Work out the finished part from the listing and answer in its coordinate system (mm). A direction names the side the tool comes from. Round coordinates to 2 decimals unless told otherwise and drop trailing zeros. Order: outer loops, then holes, each group sorted by start corner. A loop starts at its lowest first (then second) coordinate and runs counter-clockwise, first axis right, second up. Notation, with made-up numbers: (19.25, -11.5) - (42.25, -11.5) arc R29 ccw to (42.25, 11.5) - close; hole circle Ø5 at (59, 0). An arc over 180 degrees is marked (long way). One line per question, with ' | ' between items. Start each with the question number.
from build123d import *

# Parameters (mm, degrees)
BOSS_EXTRUDE2_DEPTH      = 7
BOSS_EXTRUDE4_DEPTH      = 3
BOSS_EXTRUDE4_DEPTH_BACK = 3.4
SKETCH2_W                = 10
SKETCH2_H                = 10
SKETCH3_R                = 1.5
CUT_EXTRUDE1_DEPTH       = 10
SKETCH4_W                = 8
SKETCH4_H                = 3
BOSS_EXTRUDE5_DEPTH      = 7
SKETCH5_R                = 1.5
CUT_EXTRUDE2_DEPTH       = 7
FILLET1_R                = 5
FILLET2_R                = 5
FILLET3_R                = 5
FILLET4_R                = 2
FILLET5_R                = 2
SKETCH6_W                = 30
SKETCH6_H                = 41
BOSS_EXTRUDE6_DEPTH      = 8
SKETCH7_W                = 20
SKETCH7_H                = 23
CUT_EXTRUDE3_DEPTH       = 24
SKETCH8_R                = 1.5
CUT_EXTRUDE5_DEPTH       = 54


with BuildPart() as part:
    # Sketch1 → Boss-Extrude2 (new body)
    with BuildSketch(Plane.XY):
        with BuildLine():
            Line((36, 0), (31, 0))
            ThreePointArc((31, 0), (30.997217748, -0.415321451), (30.98887149, -0.830568352))
            ThreePointArc((30.98887149, -0.830568352), (29.746163614, -2.974229152), (30.539836631, -5.321501534))
            ThreePointArc((30.539836631, -5.321501534), (0.032857513, -30.999982587), (-30.528487289, -5.386229095))
            ThreePointArc((-30.528487289, -5.386229095), (-29.731741507, -3.029439038), (-30.987456583, -0.881779181))
            ThreePointArc((-30.987456583, -0.881779181), (-30.996863987, -0.440934196), (-31, 0))
            Line((-31, 0), (-36, 0))
            ThreePointArc((-36, 0), (-30.002092566, -19.89659372), (-14.006975463, -33.163302586))
            Line((-14.006975463, -33.163302586), (-14.006975463, -72.252490852))
            Line((-14.006975463, -72.252490852), (15.993024537, -72.252490852))
            Line((15.993024537, -72.252490852), (15.993024537, -32.252490852))
            ThreePointArc((15.993024537, -32.252490852), (30.592065012, -18.976974425), (36, 0))
        make_face()
    extrude(amount=BOSS_EXTRUDE2_DEPTH)

    # Sketch2 → Boss-Extrude4 (add, two sides: drawn at the far end of the back side and taken through both)
    with BuildSketch(Plane(origin=(0, 0, 0), x_dir=(-1, 0, 0), z_dir=(0, 0, -1)).offset(-BOSS_EXTRUDE4_DEPTH_BACK)):
        with Locations((38, 0)):
            Rectangle(SKETCH2_W, SKETCH2_H)
    extrude(amount=BOSS_EXTRUDE4_DEPTH + BOSS_EXTRUDE4_DEPTH_BACK)

    # Sketch3 → Cut-Extrude1 (cut)
    with BuildSketch(Plane.XY.offset(3.4)):
        with Locations((-39, 1)):
            Circle(SKETCH3_R)
    extrude(amount=-CUT_EXTRUDE1_DEPTH, mode=Mode.SUBTRACT)

    # Sketch4 → Boss-Extrude5 (add)
    with BuildSketch(Plane(origin=(0, 0, 0), x_dir=(-1, 0, 0), z_dir=(0, 0, -1))):
        with Locations((-39, -1.5)):
            Rectangle(SKETCH4_W, SKETCH4_H)
    extrude(amount=-BOSS_EXTRUDE5_DEPTH)

    # Sketch5 → Cut-Extrude2 (cut)
    with BuildSketch(Plane.XZ.offset(3)):
        with Locations((39.374782229, 3.5)):
            Circle(SKETCH5_R)
    extrude(amount=-CUT_EXTRUDE2_DEPTH, mode=Mode.SUBTRACT)

    # Fillet1
    fillet1_edges = [part.edges().sort_by_distance(p)[0] for p in [
        (-43, -5, 0.2),
    ]]
    fillet(fillet1_edges, radius=FILLET1_R)

    # Fillet2
    fillet2_edges = [part.edges().sort_by_distance(p)[0] for p in [
        (-43, 5, 0.2),
    ]]
    fillet(fillet2_edges, radius=FILLET2_R - 0.0001)  # a hair under: the kernel refuses the full size

    # Fillet3
    fillet3_edges = [part.edges().sort_by_distance(p)[0] for p in [
        (-33, 5, 0.2),
    ]]
    fillet(fillet3_edges, radius=FILLET3_R)

    # Fillet4
    fillet4_edges = [part.edges().sort_by_distance(p)[0] for p in [
        (43, -1.5, 0),
    ]]
    fillet(fillet4_edges, radius=FILLET4_R)

    # Fillet5
    fillet5_edges = [part.edges().sort_by_distance(p)[0] for p in [
        (43, -1.5, 7),
    ]]
    fillet(fillet5_edges, radius=FILLET5_R)

    # Sketch6 → Boss-Extrude6 (add)
    with BuildSketch(Plane(origin=(0, 0, 0), x_dir=(-1, 0, 0), z_dir=(0, 0, -1))):
        with Locations((-0.993024537, -51.752490852)):
            Rectangle(SKETCH6_W, SKETCH6_H)
    extrude(amount=BOSS_EXTRUDE6_DEPTH)

    # Sketch7 → Cut-Extrude3 (cut)
    with BuildSketch(Plane(origin=(0, 0, -8), x_dir=(-1, 0, 0), z_dir=(0, 0, -1))):
        with Locations((-0.993024537, -52.752490852)):
            Rectangle(SKETCH7_W, SKETCH7_H)
    extrude(amount=-CUT_EXTRUDE3_DEPTH, mode=Mode.SUBTRACT)

    # Sketch8 → Cut-Extrude5 (cut)
    with BuildSketch(Plane(origin=(15.993024537, 0, 0), x_dir=(0, 0, -1), z_dir=(1, 0, 0))):
        with Locations(Location((0.5, -45.252490852, 0), (0, 0, 90))):
            Circle(SKETCH8_R)
        with Locations(Location((0.5, -57.252490852, 0), (0, 0, 90))):
            Circle(SKETCH8_R)
    extrude(amount=-CUT_EXTRUDE5_DEPTH, mode=Mode.SUBTRACT)


solid = part.part
1) Section C-C on x = 7 is taken. Give the vertices of the cut face in (y, z), and give its area (3 significant figures).
2) Flat-ended cylindrical pins translate along their axes: pin 1 (4.5 mm diameter, centred on y = -58, z = -4, fed in from -X); pin 2 (11 mm diameter, centred on x = -40, y = -2.5, fed in from +Z); pin 3 (1 mm diameter, centred on y = -64.5, z = 2.5, fed in from +X); pin 4 (2.5 mm diameter, centred on y = -3.5, z = -2, fed in from +X). Find the tip coordinate at first contact, or state that the pin passes through.
3) For faces 1 (the flat face through (-33, -3, -1)), 2 (the flat face through (1, -64.252, -1)), 3 (the flat face through (1, -31.252, -4)), determine the directions among +Z, -Z, +X, -X, +Y, -Y from which every point of the face is accessible in a straight line to the end or side of a thin tool.
4) Section D-D on y = -17 is taken. Give the vertices of the cut face in (x, z).
5) Straight lines are drawn through the part: line 1 (Y direction, x = -1, z = -6.5); line 2 (X direction, y = -63.5, z = -6); line 3 (X direction, y = -1, z = 3.75). For each, find the intervals that lie inside material, in ascending order.
6) Section B-B on y = 1 is taken. Give the vertices of the cut face in (x, z).
7) Section A-A on z = -6.5 is taken. Give the vertices of the cut face in (x, y).
8) Determine the mould class of faces 4 (the cylindrical face through (-42, 3, 0)), 5 (the cylindrical face through (-11.472, -55.867, -1.075)), 6 (the cylindrical face through (0.639, -30.993, 3.451)), 7 (the flat face through (43, -2, 3)) for opening direction X: released by +X, released by -X, zero draft, split by the parting line, or undercut.
Recorded:
1) outline: (-72.25, -8) - (-64.25, -8) - (-64.25, 7) - (-72.25, 7) - close; (-41.25, -8) - (-31.25, -8) - (-31.25, 0) - (-30.2, 0) - (-30.2, 7) - (-41.25, 7) - close | area: 277 mm²
2) pin 1: stops at x = -14.01 | pin 2: stops at z = 7 | pin 3: stops at x = 15.99 | pin 4: stops at x = -33
3) face 1: -Z, +X, +Y, -Y | face 2: +Z, -Z | face 3: -Z, +X, -X, +Y
4) outline: (-31.73, 0) - (-25.92, 0) - (-25.92, 7) - (-31.73, 7) - close; (25.92, 0) - (31.73, 0) - (31.73, 7) - (25.92, 7) - close
5) line 1: y = -72.25 to -64.25, -41.25 to -31.25 | line 2: x = -14.01 to -9.01, 10.99 to 15.99 | line 3: x = -35.99 to -30.83, 30.77 to 37.9, 40.85 to 43
6) outline: (-42.9, -3) - (-40.5, -3) - (-40.5, 3.4) - (-42.9, 3.4) - close; (-37.5, -3) - (-33.1, -3) - (-33.1, 3.4) - (-37.5, 3.4) - close
7) outline: (-14.01, -72.25) - (15.99, -72.25) - (15.99, -31.25) - (-14.01, -31.25) - close; hole (-9.01, -64.25) - (10.99, -64.25) - (10.99, -41.25) - (-9.01, -41.25) - close
8) face 4: released by -X | face 5: zero draft | face 6: undercut | face 7: released by +X
